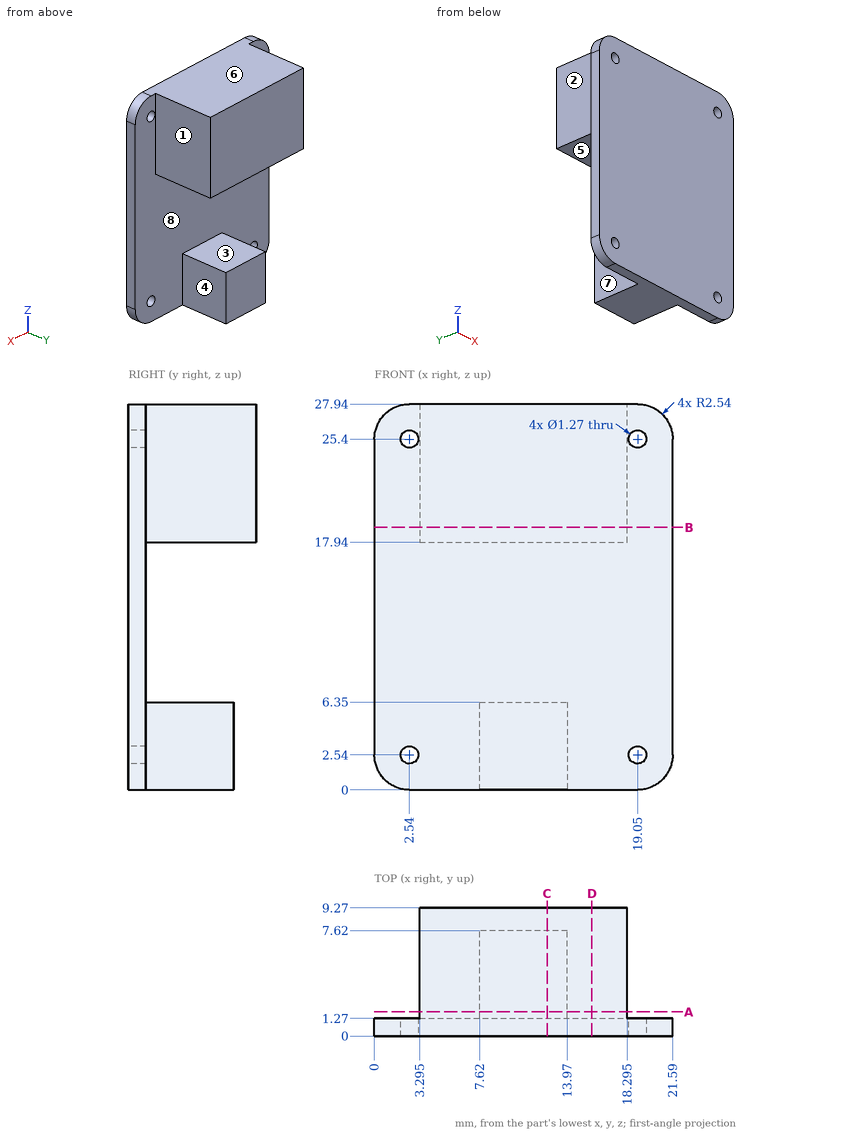
Study the drawing (mm; zero at the part's minimum x, y, z) and answer. A direction names the side the tool comes from. Coordinates: 2 decimals unless noted, no trailing zeros. Order: outer loops, then holes, each group sorted by start corner. A loop starts at its lowest first (then second) coordinate and runs counter-clockwise, first axis right, second up. Notation, with made-up numbers: (41, -10.75) -> (87, -10.75) arc R26 ccw to (87, 17.25) -> close; hole circle Ø4 at (20, 80.25). An arc over 180 degrees is marked (long way). Answer in a Markdown table with one row per item. Add a question column.
Item 1: Each of these flat-tipped pins is pushed along its axis until it touches: P1, Ø4, axis at y = 6.5, z = 21, coming from the +X side (3 decimals); P2, Ø4, axis at y = 6, z = 20.5, coming from the -X side (3 decimals); P3, Ø7, axis at x = 12.5, z = 4.5, coming from the +Y side; P4, Ø0.8, axis at x = 2.54, z = 25.4, coming from the -Y side. Where does it stop, or does it pass through?
Item 2: Find section B-B (z = 19). Write down the section's boundary in (x, y) (3 decimals).
Item 3: Find section C-C (x = 12.5). Write down the section's boundary in (y, z).
Item 4: Find section D-D (x = 15.75). Write down the section's boundary in (y, z), then the cut area to 3 significant figures.
Item 5: Determine the mould class of the marked faces 5, 6, 7 and 8 for opening direction Z: +Z half, -Z half, draft (parallel to the pull), parting line (faces both ways), or undercut.
Item 6: Find the intervals of material crossed by L1, parallel to Z at x = 2.54, y = 0.85 (3 decimals); L2, parallel to Z at x = 7.75, y = 3.5; L3, parallel to X at y = 0.5, z = 25, in increasing order. Write a range as from..to.
Item 7: Find section A-A (y = 1.75). Write down the section's boundary in (x, z) (3 decimals), then the cut area to 3 significant figures.
Item 8: Which of the six approach directions +Z, -Z, +X, -X, +Y, -Y give full straight-line access (tool end or side, diameter ignored) to the marked faces 1, 2, 3 and 4?
Result set:
| question | item | result |
|---|---|---|
| 1 | P1 | stops at x = 18.295 |
| 1 | P2 | stops at x = 3.295 |
| 1 | P3 | stops at y = 7.62 |
| 1 | P4 | passes through |
| 2 | outline | (0, 0) -> (21.59, 0) -> (21.59, 1.27) -> (18.295, 1.27) -> (18.295, 9.27) -> (3.295, 9.27) -> (3.295, 1.27) -> (0, 1.27) -> close |
| 3 | outline | (0, 0) -> (7.62, 0) -> (7.62, 6.35) -> (1.27, 6.35) -> (1.27, 17.94) -> (9.27, 17.94) -> (9.27, 27.94) -> (0, 27.94) -> close |
| 4 | outline | (0, 0) -> (1.27, 0) -> (1.27, 17.94) -> (9.27, 17.94) -> (9.27, 27.94) -> (0, 27.94) -> close |
| 4 | area | 115 mm² |
| 5 | face 5 | undercut |
| 5 | face 6 | +Z half |
| 5 | face 7 | draft |
| 5 | face 8 | undercut |
| 6 | L1 | z = 0..1.905, 3.175..24.765, 26.035..27.94 |
| 6 | L2 | z = 0..6.35, 17.94..27.94 |
| 6 | L3 | x = 0..2.05, 3.03..18.56, 19.54..21.59 |
| 7 | outline | (3.295, 17.94) -> (18.295, 17.94) -> (18.295, 27.94) -> (3.295, 27.94) -> close; (7.62, 0) -> (13.97, 0) -> (13.97, 6.35) -> (7.62, 6.35) -> close |
| 7 | area | 190 mm² |
| 8 | face 1 | +Z, -Z, +X, +Y |
| 8 | face 2 | +Z, -Z, -X, +Y |
| 8 | face 3 | +X, -X, +Y |
| 8 | face 4 | -Z, +X, +Y |
